Autodesk Inventor part; units mm, degrees
ref_plane "Work Plane1" through (65.1649, 36.0099, -59.025) normal (0, 0, -1) x (0, -1, 0)
ref_plane "Work Plane2" through (0, 0, 0) normal (0, 0, 1) x (1, 0, 0)
ref_plane "YZ Plane" through (0, 0, 0) normal (1, 0, 0) x (0, 1, 0)
ref_plane "Work Plane1" through (65.1649, 36.0099, -59.025) normal (0, 0, -1) x (0, -1, 0)
ref_plane "Work Plane2" through (0, 0, 0) normal (0, 0, 1) x (1, 0, 0)
sketch "Sketch1" plane through (0, 0, 0) normal (0, 0, 1) x (1, 0, 0)
  line L0 (27.0649, 36.0099) -> (65.1649, 36.0099) construction
  line L1 (-10, 0) -> (-10, 27.6599) construction
  line L2 (102.2297, 27.6599) -> (102.2297, 0) construction
  line L3 (89.2297, 29.6599) -> (100.2297, 29.6599) construction
  line L4 (-10, 36.0099) -> (102.2297, 36.0099)
  line L5 (102.2297, 36.0099) -> (102.2297, 29.6599)
  line L6 (92.075, 29.6599) -> (-10, 29.6599)
  line L7 (-10, 29.6599) -> (-10, 36.0099)
  line L8 (92.075, 29.6599) -> (92.075, 16.9599)
  line L9 (92.075, 16.9599) -> (102.2297, 16.9599)
  line L10 (102.2297, 16.9599) -> (102.2297, 29.6599)
  circle A0 centre (97.2297, 24.6599) radius 1.965
  circle A1 centre (97.2297, 24.6599) radius 1.965 construction
  point P0 (0, 0)
extrude "Extrusion1" add sketch "Sketch1" along normal blind 7.366
fillet "Fillet1" radius 3.175 4 edges at (92.075, 29.6599, 3.683) (102.2297, 36.0099, 3.683) (92.075, 16.9599, 3.683) (102.2297, 16.9599, 3.683)
sketch "Sketch2" plane through (0, 0, 0) normal (0, 0, -1) x (-1, 0, 0)
  line L0 (10, 0) -> (10, 27.6599) construction
  line L1 (-88.9, 29.6599) -> (10, 29.6599)
  line L2 (10, 29.6599) -> (-6.51, 29.6599)
  line L3 (-6.51, 29.6599) -> (-6.51, 22.0399)
  line L4 (-6.51, 22.0399) -> (10, 22.0399)
  line L5 (10, 22.0399) -> (10, 29.6599)
  point P0 (0, 0)
  dimension "d4" = 16.51
  dimension "d5" = 7.62
extrude "Extrusion2" add sketch "Sketch2" against normal blind 1.27
fillet "Fillet2" radius 1.524 1 edges at (-1.745, 29.6599, 1.27)
sketch "Sketch3" plane through (0, 0, 0) normal (0, 0, -1) x (-1, 0, 0)
  circle A0 centre (5, 24.6599) radius 1.965 construction
  arc A1 (6.8415, 24.6599) -> (3.1585, 24.6599) centre (5, 24.6599) ccw
  line L0 (3.1585, 24.6599) -> (6.8415, 24.6599)
  point P0 (0, 0)
  dimension "d9" = 3.683
revolve "Revolution1" add sketch "Sketch3" angle 180 about axis through (-3.1585, 24.6599, 0) along (-1, 0, 0)
sketch "Sketch4" plane through (-10, 29.6599, 7.366) normal (0, -1, 0) x (1, 0, 0)
  line L0 (37.0649, -133.32) -> (37.0649, 0.03) construction
  line L1 (75.1649, 0.03) -> (75.1649, -133.32) construction
  line L2 (0, 0) -> (98.9, 0) construction
  line L3 (109.0547, 0) -> (0, 0) construction
  line L4 (37.0649, 0) -> (37.0649, -7.366) construction
  line L5 (0, -7.366) -> (109.0547, -7.366) construction
  line L6 (75.1649, 0) -> (75.1649, -7.366) construction
  line L7 (37.0649, -3.683) -> (75.1649, -3.683) construction
  point P0 (10, -7.366)
  point P1 (42.1449, -3.683)
  point P2 (70.0849, -3.683)
  dimension "d11" = 5.08
  dimension "d12" = 5.08
hole "Hole1" at (32.1449, 29.6599, 3.683) at (60.0849, 29.6599, 3.683) direction (0, 1, 0) diameter 3.937 end through all
fillet "Fillet3" radius 3.175 1 edges at (-10, 36.0099, 3.683)
fillet "Fillet4" radius 1.524 1 edges at (6.51, 29.6599, 1.397)
properties part number "PhoneMountRightRib"
The model under review builds one solid part; all positions refer to its coordinate system, in mm. A direction names the side the tool comes from. Round coordinates to 2 decimals unless told otherwise and drop trailing zeros. Order: outer loops, then holes, each group sorted by start corner. A loop starts at its lowest first (then second) coordinate and runs counter-clockwise, first axis right, second up. Notation, with made-up numbers: (-1, -13.75) -> (43, -13.75) arc R32 ccw to (43, 21.25) -> close; hole circle Ø8 at (2, -31.75). An arc over 180 degrees is marked (long way). Use CSV: the item, a comma, the result in double quotes. Start each with the question number.
(1) Mouldability with a two-part tool opening along Z and no side actions: class faces 4 (the face through (34.067, 32.879, 4.11)), 5 (the face through (47, 31, 0)), 6 (the face through (-10, 30, 3)) as pulls with the +Z half, pulls with the -Z half, needs draft (parallel to the pull), parting line crosses it, or undercut.
(2) Wall thickness on probe 1 along Y at (x, z) = (97, 3.25); probe 2 along X at (y, z) = (29.75, 2.25); probe 3 along X at (y, z) = (29.75, 4): over which ranges is each line inside the solid? List them lowest first. Write a range as from..to.
(3) Consider section D-D on y = 18.5. Write out the cut boundary in (x, z).
(4) Consider section A-A on z = 4.25. Write out the cut boundary in (x, y) (3 decimals), and give its area (3 significant figures).
(5) Consider section B-B on x = -2. Write out the cut boundary in (y, z).
(6) Tool access review of faces 1 (the face through (91.17, 28.705, 3.735)), 2 (the face through (-2, 25, 1.27)), 3 (the face through (40, 29.66, 4)): name each direction out of +Z, -Z, +X, -X, +Y, -Y from which nothing blocks a thin tool from reaching the whole face with its end or side.
(7) Insertion check: pin 1 (2 mm diameter, centred on x = 52.5, z = 3, fed in from -Y); pin 2 (5 mm diameter, centred on x = 74.5, y = 32.5, fed in from -Z); pin 3 (3 mm diameter, centred on x = 60.08, z = 3.68, fed in from -Y); pin 4 (1.9 mm diameter, centred on y = 22, z = 3, fed in from -X) (3 decimals). Each pin has a flat end and moves straight along its axis. Give the tip position at first contact, or say it passes through.
(8) Consider section C-C on y = 31.5. Write out the cut boundary in (x, z).
Responses:
1,face 4,"undercut"
1,face 5,"pulls with the -Z half"
1,face 6,"needs draft"
2,probe 1,"16.96..22.71, 26.61..36.01"
2,probe 2,"-10..30.8, 33.49..58.74, 61.43..102.23"
2,probe 3,"-10..30.2, 34.09..58.14, 62.03..102.23"
3,outline,"(92.53, 0) -> (101.78, 0) -> (101.78, 7.37) -> (92.53, 7.37) -> close"
4,outline,"(-10, 29.66) -> (30.26, 29.66) -> (30.26, 36.01) -> (-6.825, 36.01) arc R3.175 ccw to (-10, 32.835) -> close; (34.03, 29.66) -> (58.2, 29.66) -> (58.2, 36.01) -> (34.03, 36.01) -> close; (61.97, 29.66) -> (88.9, 29.66) arc R3.175 cw to (92.075, 26.485) -> (92.075, 20.135) arc R3.175 ccw to (95.25, 16.96) -> (99.055, 16.96) arc R3.175 ccw to (102.23, 20.135) -> (102.23, 32.835) arc R3.175 ccw to (99.055, 36.01) -> (61.97, 36.01) -> close; hole circle Ø3.93 at (97.23, 24.66)"
4,area,"775 mm²"
5,outline,"(22.04, 0) -> (36.01, 0) -> (36.01, 7.37) -> (29.66, 7.37) -> (29.66, 2.79) arc R1.52 cw to (28.14, 1.27) -> (22.04, 1.27) -> close"
6,face 1,"+Z, -Z, -Y"
6,face 2,"+Z, -X, -Y"
6,face 3,"+Z, -Y"
7,pin 1,"y = 29.66"
7,pin 2,"z = 0"
7,pin 3,"through"
7,pin 4,"x = 92.075"
8,outline,"(-10, 0) -> (102.23, 0) -> (102.23, 7.37) -> (-10, 7.37) -> close; hole circle Ø3.94 at (32.14, 3.68); hole circle Ø3.94 at (60.08, 3.68)"
